from build123d import *

# Parameters (mm, degrees)
F0_W     = 155.6676864983
F0_H     = 89.0193315694
F1_DEPTH = 82.042
F2_R     = 12.7
F3_R     = 5.08
F4_T     = -7.62


with BuildPart() as f1:
    # F0 (on Front) → F1 (new body, symmetric)
    with BuildSketch(Plane.XZ):
        with Locations((63.3336471573, 10.4723514293)):
            Rectangle(F0_W, F0_H)
    extrude(amount=F1_DEPTH, both=True)

    # F2
    f2_edges = [f1.edges().sort_by_distance(p)[0] for p in [
        (-14.500196, 0, 54.982017),
        (-14.500196, 0, -34.037314),
        (141.16749, 0, 54.982017),
        (141.16749, 0, -34.037314),
    ]]
    fillet(f2_edges, radius=F2_R)

    # F3
    f3_edges = [f1.edges().sort_by_distance(p)[0] for p in [
        (-10.780452, 82.042, -30.31757),
    ]]
    fillet(f3_edges, radius=F3_R)

    # F4
    f4_openings = [f1.faces().sort_by_distance(p)[0] for p in [
        (63.333647, -82.042, 10.472351),
    ]]
    offset(amount=F4_T, openings=f4_openings)


solid = f1.part
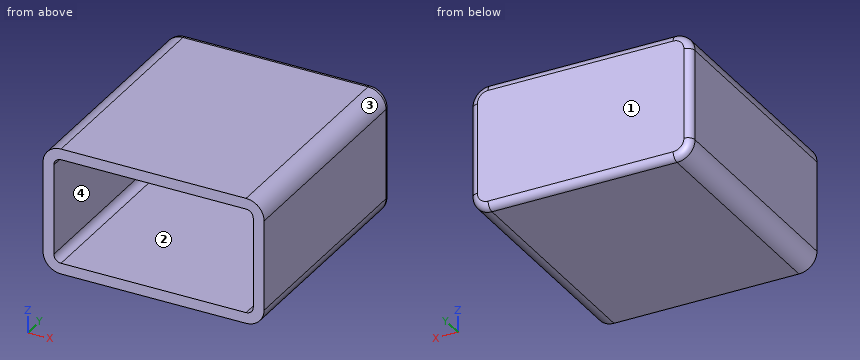
Geometry check sheet. Reference: the model listing, model coordinates, mm. Face numbers are marked on the shaded views. Coordinates: 2 decimals unless noted, no trailing zeros. Order: outer loops, then holes, each group sorted by start corner. A loop starts at its lowest first (then second) coordinate and runs counter-clockwise, first axis right, second up. Notation, with made-up numbers: (42, 34) - (69, 34) arc R12 cw to (69, 45) - close; hole circle Ø11 at (23, 25.5). An arc over 180 degrees is marked (long way). Answer in a Markdown table with one row per item. Add a question column.
1) Cross-section at C-C, the plane x = 13. Record the cut outline in (y, z), then the cut area to 3 significant figures.
2) Cross-section at A-A, the plane z = -4. Record the cut outline in (x, y), then the cut area to 3 significant figures.
3) Material ranges on line 1 along X through (y, z) = (-49, 34.5); line 2 along Z through (x, y) = (12, 59); line 3 along Y through (x, z) = (98.5, -21), recorded low to high. Write a range as [from, to].
4) Cross-section at B-B, the plane y = -67.5. Record the cut outline in (x, z), then the cut area to 3 significant figures.
5) Release check for a two-part mould opening along Z. For the marked faces 1, 2, 3 and 4 record: +Z half, -Z half, draft (parallel to the pull), parting line (faces both ways), or undercut.
Check result:
| question | item | result |
|---|---|---|
| 1 | outline | (-82.04, -34.04) - (76.96, -34.04) arc R5.08 ccw to (82.04, -28.96) - (82.04, 49.9) arc R5.08 ccw to (76.96, 54.98) - (-82.04, 54.98) - (-82.04, 47.36) - (74.42, 47.36) - (74.42, -26.42) - (-82.04, -26.42) - close |
| 1 | area | 3,050 mm² |
| 2 | outline | (-14.5, -82.04) - (-6.88, -82.04) - (-6.88, 74.42) - (133.55, 74.42) - (133.55, -82.04) - (141.17, -82.04) - (141.17, 76.96) arc R5.08 ccw to (136.09, 82.04) - (-9.42, 82.04) arc R5.08 ccw to (-14.5, 76.96) - close |
| 2 | area | 3,560 mm² |
| 3 | line 1 | x = [-14.5, -6.88], [133.55, 141.17] |
| 3 | line 2 | z = [-34.04, -26.42], [47.36, 54.98] |
| 3 | line 3 | y = [74.42, 82.04] |
| 4 | outline | (-14.5, -21.34) arc R12.7 ccw to (-1.8, -34.04) - (128.47, -34.04) arc R12.7 ccw to (141.17, -21.34) - (141.17, 42.28) arc R12.7 ccw to (128.47, 54.98) - (-1.8, 54.98) arc R12.7 ccw to (-14.5, 42.28) - close; hole (-6.88, -21.34) arc R5.08 ccw to (-1.8, -26.42) - (128.47, -26.42) arc R5.08 ccw to (133.55, -21.34) - (133.55, 42.28) arc R5.08 ccw to (128.47, 47.36) - (-1.8, 47.36) arc R5.08 ccw to (-6.88, 42.28) - close |
| 4 | area | 3,380 mm² |
| 5 | face 1 | draft |
| 5 | face 2 | undercut |
| 5 | face 3 | +Z half |
| 5 | face 4 | undercut |
